Read the model definition and answer for the solid it produces. Units are mm, in the model's axes. Face numbers are marked on the shaded views. A direction names the side the tool comes from. Coordinates: 2 decimals unless noted, no trailing zeros. Order: outer loops, then holes, each group sorted by start corner. A loop starts at its lowest first (then second) coordinate and runs counter-clockwise, first axis right, second up. Notation, with made-up numbers: (16.5, 76.5) - (68.5, 76.5) arc R15 cw to (68.5, 104.5) - close; hole circle Ø4 at (20.25, 57.5). An arc over 180 degrees is marked (long way). Write item = value, one per line.
Autodesk Inventor part; units mm, degrees
ref_plane "YZ Plane" through (0, 0, 0) normal (1, 0, 0) x (0, 1, 0)
ref_plane "XZ Plane" through (0, 0, 0) normal (0, 1, 0) x (-1, 0, 0)
ref_plane "XY Plane" through (0, 0, 0) normal (0, 0, 1) x (1, 0, 0)
sketch "Sketch1" plane through (0, 0, 0) normal (0, 0, 1) x (1, 0, 0)
  circle A0 centre (91.35, 6.3991) radius 1.6
  circle A1 centre (70.85, 18.1613) radius 2.25
  circle A2 centre (91.35, 6.3991) radius 3
  line L0 (76.4305, 15.9113) -> (89.3317, 4.1796)
  line L1 (78.8117, 18.6299) -> (93.0461, 8.8737)
  circle A3 centre (70.85, 13.6613) radius 1.6
  circle A4 centre (70.85, 18.1613) radius 1.625
  line L2 (76.4305, 15.9113) -> (70.85, 15.9113)
  line L3 (78.8117, 18.6299) -> (72.5761, 19.6046)
  point P0 (0, 0)
  point P1 (72.1824, 12.7754)
  point P2 (69.5176, 12.7754)
  dimension "d0" = 4.5
  dimension "d1" = 6
extrude "Extrusion1" add sketch "Sketch1" along normal mid plane 4 contours A1 | A1 L3 L1 A2 L0 L2 | A2
properties part number "Palanca metacarpo_distal"
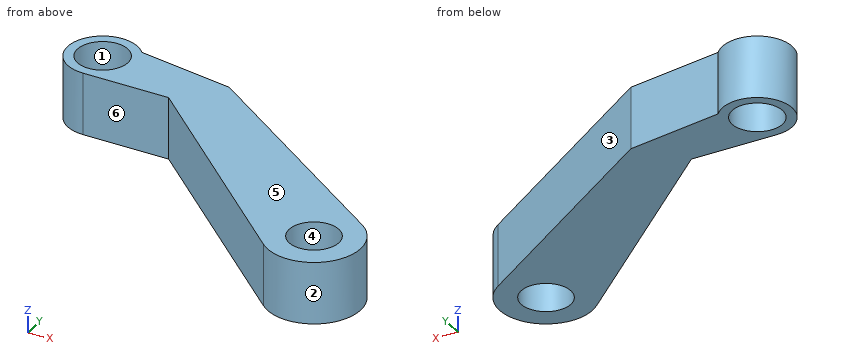
1) For the marked faces 5 and 6, determine the directions among +Z, -Z, +X, -X, +Y, -Y from which every point of the face is accessible in a straight line to the end or side of a thin tool.
Returned:
face_5 = +Z, +X, -X, +Y, -Y
face_6 = +Z, -Z, -X, -Y
2) Straight lines are drawn through the part: line 1 along Y through (x, z) = (70.85, -0.7); line 2 along X through (y, z) = (6.25, -0.55); line 3 along Y through (x, z) = (71.75, 1.45). For each, find the intervals that lie inside material, in ascending order. Write a range as from..to.
Returned:
line_1 = 15.91..16.54, 19.79..20.41
line_2 = 87.05..89.76, 92.94..94.35
line_3 = 15.91..16.81, 19.51..20.22
3) The part is cut by section B-B (x = 91.35). Determine the outline of the cut face in (y, z).
Returned:
outline = (3.4, -2) - (4.8, -2) - (4.8, 2) - (3.4, 2) - close; (8, -2) - (10.04, -2) - (10.04, 2) - (8, 2) - close
4) Determine the mould class of the marked faces 1, 2, 3 and 4 for opening direction X: pulls with the +X half, pulls with the -X half, needs draft (parallel to the pull), parting line crosses it, or undercut.
Returned:
face_1 = undercut
face_2 = parting line crosses it
face_3 = pulls with the +X half
face_4 = undercut
5) Flat-ended cylindrical pins translate along their axes: pin 1 Ø1.5 at (x, z) = (75.5, 0.5) entering from -Y; pin 2 Ø10 at (x, y) = (88.5, 15.5) entering from -Z; pin 3 Ø2 at (x, z) = (81.5, 0) entering from +Y; pin 4 Ø3 at (x, y) = (91.35, 6.4) entering from -Z. Find the tip coordinate at first contact, or state that the pin passes through.
Returned:
pin_1 = 15.91
pin_2 = -2
pin_3 = 17.47
pin_4 = through
6) The part is cut by section C-C (z = 0.8). Count the separate pieces of the cut face and the enclosed holes in it, and give its area (3 significant figures).
Returned:
separate_pieces = 1
enclosed_holes = 2
area = 114 mm^2
7) The part is cut by section A-A (y = 17.5). Determine the outline of the cut face in (x, z), and give its area (3 significant figures).
Returned:
outline = (68.7, -2) - (69.37, -2) - (69.37, 2) - (68.7, 2) - close; (72.33, -2) - (80.46, -2) - (80.46, 2) - (72.33, 2) - close
area = 35.2 mm^2
8) The part is cut by section D-D (y = 11.5). Determine the outline of the cut face in (x, z), and give its area (3 significant figures).
Returned:
outline = (81.28, -2) - (89.21, -2) - (89.21, 2) - (81.28, 2) - close
area = 31.7 mm^2
